Input: dimensioned drawing with shaded views. Units: mm. Origin: part minimum x, y, z. A direction names the side the tool comes from. Round coordinates to 2 decimals unless told otherwise and drop trailing zeros. Loops run counter-clockwise (first coordinate to the right, second up) from the corner with the lowest first, then second, coordinate; pieces in that order, holes last. Notation, with made-up numbers: M 42,85.5 L 51,85.5 A24 ccw 51,95.5 Z; hole C 78.25,82 d2. An arc over 180 degrees is marked long. Write each question's results on one line, items separated by ' | '. Start each with the question number.
1. Section A-A on y = 10. Output: boundary loops of the cut face in (x, z).
2. Set-up query: the marked faces 3, 4, 5 and 6. Return all of +Z, -Z, +X, -X, +Y, -Y with unobstructed straight access to the full face (end or side cutting, diameter ignored); none if empty.
3. Section C-C on z = 8.5. Output: boundary loops of the cut face in (x, y).
4. Contact query for flat-ended pins moving along their axis: pin 1 Ø3 at (x, z) = (3.5, 15.5) entering from +Y (3 decimals); pin 2 Ø4 at (x, y) = (15, 7.5) entering from +Z; pin 3 Ø6 at (x, y) = (16.5, 9) entering from +Z. Output: stop coordinate, or through.
5. Ray query, line 1 (Y direction, x = 10, z = 23.2); line 2 (Z direction, x = 19, y = 12); line 3 (Z direction, x = 16, y = 16.5). Return the intervals inside material, ascending.
6. Section D-D on x = 2.5. Output: boundary loops of the cut face in (y, z), and give its area (3 significant figures).
7. Draft query along Y for the marked faces 1 and 2. Return one class per face: released by +Y, released by -Y, zero draft, split by the parting line, or undercut.
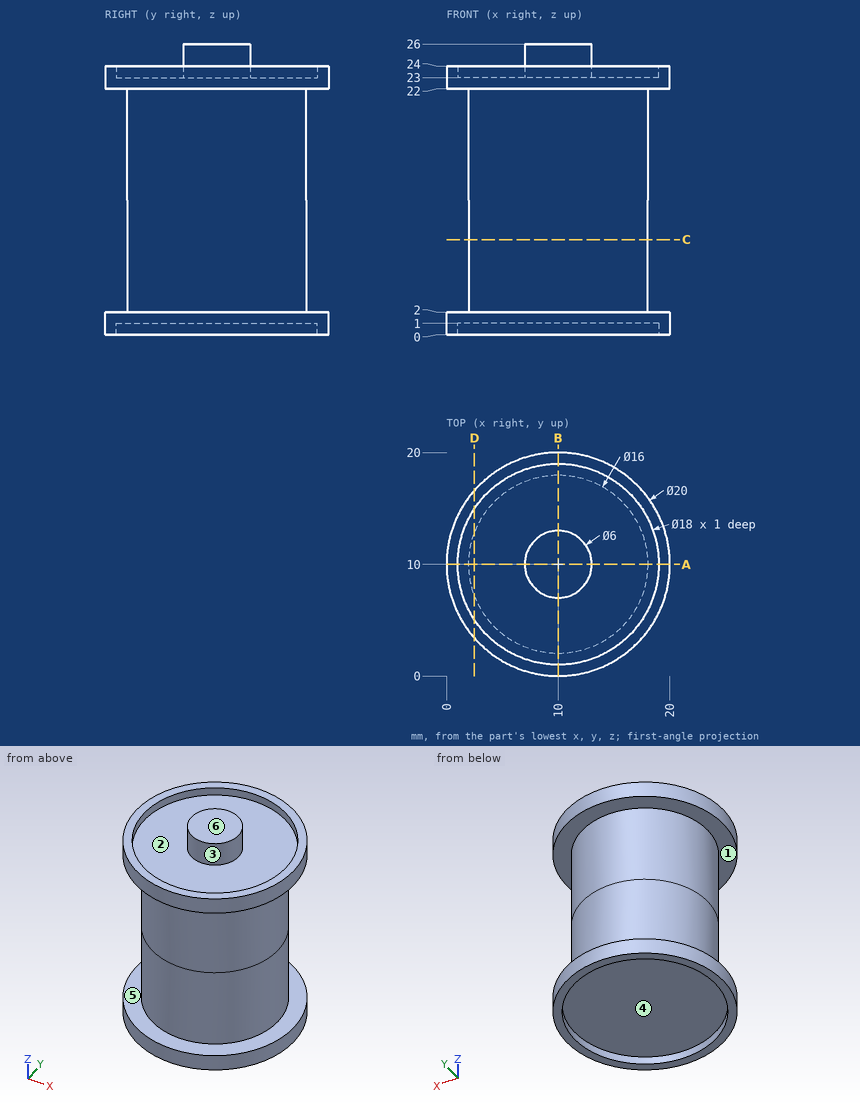
Taken from the geometry:
1) outline: M 0,0 L 1,0 L 1,1 L 19,1 L 19,0 L 20,0 L 20,2 L 18,2 L 18,22 L 20,22 L 20,24 L 19,24 L 19,23 L 13,23 L 13,26 L 7,26 L 7,23 L 1,23 L 1,24 L 0,24 L 0,22 L 2,22 L 2,2 L 0,2 Z
2) face 3: +Z | face 4: -Z | face 5: none | face 6: +Z, +X, -X, +Y, -Y
3) outline: C 10,10 d16
4) pin 1: y = 16.245 | pin 2: z = 23 | pin 3: z = 24
5) line 1: 0 to 1, 7 to 13, 19 to 20 | line 2: 0 to 2, 22 to 24 | line 3: 1 to 2, 22 to 23
6) outline: M 3.39,0 L 5.03,0 L 5.03,1 L 14.97,1 L 14.97,0 L 16.61,0 L 16.61,2 L 12.78,2 L 12.78,22 L 16.61,22 L 16.61,24 L 14.97,24 L 14.97,23 L 5.03,23 L 5.03,24 L 3.39,24 L 3.39,22 L 7.22,22 L 7.22,2 L 3.39,2 Z | area: 144 mm^2
7) face 1: zero draft | face 2: undercut
